The drawing under review shows one solid part. Ordinate dimensions are in mm from its lowest x, y, z. Coordinates: 2 decimals unless noted, no trailing zeros. Order: outer loops, then holes, each group sorted by start corner. A loop starts at its lowest first (then second) coordinate and runs counter-clockwise, first axis right, second up.
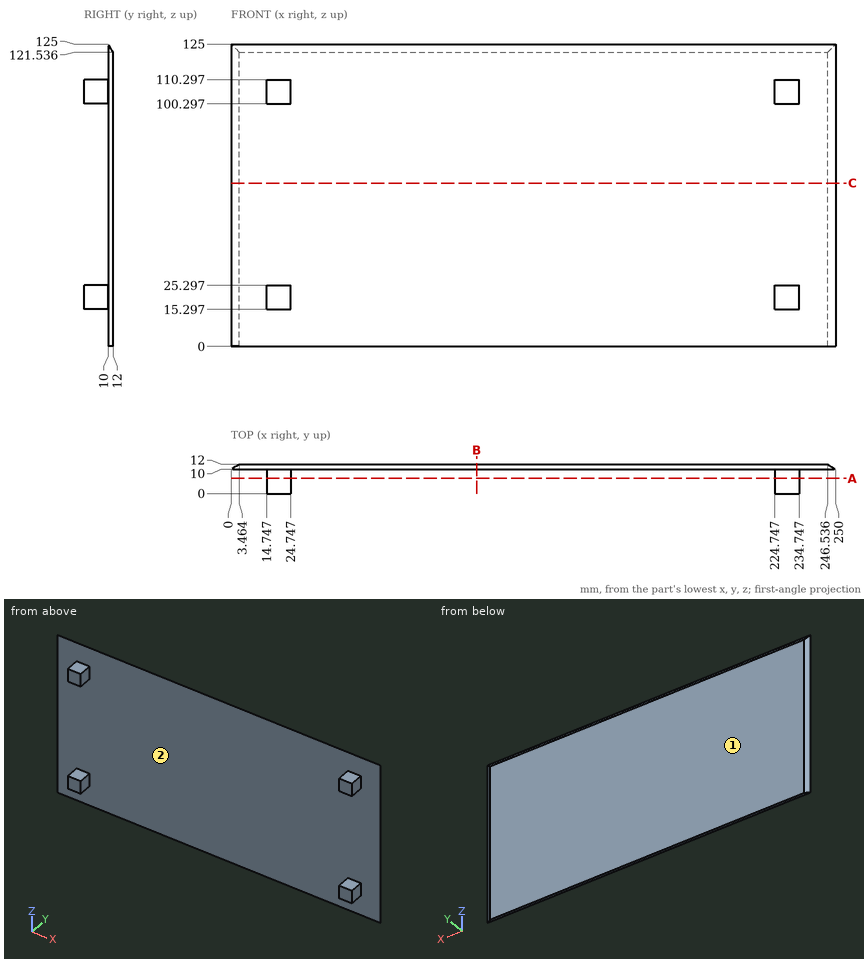
(1) Wall thickness on line 1 (Z direction, x = 232.5, y = 5.5); line 2 (X direction, y = 4.25, z = 106); line 3 (Y direction, x = 124, z = 72): over which ranges is each line inside the solid? List them lowest first.
(2) Consider section B-B (x = 101.5). Give the boundary of the cut face in (y, z).
(3) Consider section A-A (y = 6.25). Give the boundary of the cut face in (x, z).
(4) The part is to be moulded in two halves that separate along X. For the marked faces 1 and 2, say which applies: +X half, -X half, draft (parallel to the pull), parting line (faces both ways), or undercut.
(5) Insertion check: pin 1 Ø5 at (y, z) = (2.5, 107) entering from -X; pin 2 Ø5 at (y, z) = (2.5, 15) entering from +X; pin 3 Ø3 at (x, y) = (19.5, 3.5) entering from +Z. Each pin has a flat end and moves straight along its axis. Give the tip position at first contact, or say it passes through.
(6) Consider section C-C (z = 67.5). Give the boundary of the cut face in (x, y).
Findings:
1. line 1: z = 15.3 to 25.3, 100.3 to 110.3
1. line 2: x = 14.75 to 24.75, 224.75 to 234.75
1. line 3: y = 10 to 12
2. outline: (10, 0) - (12, 0) - (12, 121.54) - (10, 125) - close
3. outline: (14.75, 15.3) - (24.75, 15.3) - (24.75, 25.3) - (14.75, 25.3) - close; (14.75, 100.3) - (24.75, 100.3) - (24.75, 110.3) - (14.75, 110.3) - close; (224.75, 15.3) - (234.75, 15.3) - (234.75, 25.3) - (224.75, 25.3) - close; (224.75, 100.3) - (234.75, 100.3) - (234.75, 110.3) - (224.75, 110.3) - close
4. face 1: draft
4. face 2: undercut
5. pin 1: stops at x = 14.75
5. pin 2: stops at x = 234.75
5. pin 3: stops at z = 110.3
6. outline: (0, 10) - (250, 10) - (246.54, 12) - (3.46, 12) - close
